```python
from build123d import *

# Parameters (mm, degrees)
F1_DEPTH = 30
F2_R     = 4.4
F3_R     = 4.4
F4_DEPTH = 25
F5_R     = 2
F6_R     = 2


# Not quite as in the source:
# - a feature names something its author has since deleted; it is built from what else it names


with BuildPart() as f1:
    # F0 (on Front) → F1 (new body)
    with BuildSketch(Plane.XZ):
        Polygon((90, -1), (90, 1), (70, 1), (70, 34), (-70, 34), (-70, 1), (-90, 1), (-90, -1), (-68, -1), (-68, 32), (68, 32), (68, -1), align=None)
    extrude(amount=F1_DEPTH)

    # F2 (on face) + F3 (on face) → F4 (cut)
    with BuildSketch(Plane.XY.offset(1)):
        with Locations((-80, -15)):
            Circle(F2_R)
        with Locations((80, -15)):
            Circle(F2_R)
    with BuildSketch(Plane.XY.offset(34)):
        with Locations((-25, -15)):
            Circle(F3_R)
        with Locations((25, -15)):
            Circle(F3_R)
    extrude(amount=-F4_DEPTH, mode=Mode.SUBTRACT)

    # F5
    f5_edges = [f1.edges().sort_by_distance(p)[0] for p in [
        (-70, -15, 34),
        (70, -15, 34),
    ]]
    fillet(f5_edges, radius=F5_R)

    # F6
    f6_edges = [f1.edges().sort_by_distance(p)[0] for p in [
        (68, -15, -1),
        (-68, -15, -1),
    ]]
    fillet(f6_edges, radius=F6_R)


solid = f1.part
```
The model under review builds one solid part; all positions refer to its coordinate system, in mm. A direction names the side the tool comes from. Round coordinates to 2 decimals unless told otherwise and drop trailing zeros. Order: outer loops, then holes, each group sorted by start corner. A loop starts at its lowest first (then second) coordinate and runs counter-clockwise, first axis right, second up.
(1) Take a section at C-C, the plane y = -7.75. State the section outline as (x, z) points, plus the area to 3 significant figures.
Working result:
outline: (-90, -1) - (-70, -1) arc R2 ccw to (-68, 1) - (-68, 32) - (68, 32) - (68, 1) arc R2 ccw to (70, -1) - (90, -1) - (90, 1) - (70, 1) - (70, 32) arc R2 ccw to (68, 34) - (-68, 34) arc R2 ccw to (-70, 32) - (-70, 1) - (-90, 1) - close
area: 489 mm2
(2) Take a section at B-B, the plane z = 12.5. State the section outline as (x, y) points.
Working result:
outline: (-70, -30) - (-68, -30) - (-68, 0) - (-70, 0) - close; (68, -30) - (70, -30) - (70, 0) - (68, 0) - close
(3) Tool access review of faces 4 (the face through (85, -15, 1)), 5 (the face through (-85, -15, -1)), 6 (the face through (27.365, -11.29, 33.014)), 7 (the face through (-75, -15, 1)), 8 (the face through (-1, -15, 32)): name each direction out of +Z, -Z, +X, -X, +Y, -Y from which nothing blocks a thin tool from reaching the whole face with its end or side.
Working result:
face 4: +Z, +X, +Y, -Y
face 5: -Z, +X, -X, +Y, -Y
face 6: +Z, -Z
face 7: +Z, -X, +Y, -Y
face 8: -Z, +Y, -Y
(4) Mouldability with a two-part tool opening along Y and no side actions: class faces 1 (the face through (70, -15, 16)), 2 (the face through (0, -30, 33)), 3 (the face through (75.604, -14.807, 0.014)) as released by +Y, released by -Y, zero draft, split by the parting line, or undercut.
Working result:
face 1: zero draft
face 2: released by -Y
face 3: undercut
(5) Wall thickness on L1, parallel to Y at x = 25, z = 33.05; L2, parallel to X at y = -5.5, z = 28.5; L3, parallel to X at y = -12.5, z = 32.5: over which ranges is each line inside the solid? List them lowest first.
Working result:
L1: y = -30 to -19.4, -10.6 to 0
L2: x = -70 to -68, 68 to 70
L3: x = -69.94 to -28.62, -21.38 to 21.38, 28.62 to 69.94
(6) For P1, Ø6, axis at y = -6.5, z = 29, coming from the +X side; P2, Ø5, axis at x = 49, y = -14, coming from the -Z side; P3, Ø10, axis at x = -80, y = -15, coming from the +Z side, all flat-tipped, find the tip position at first contact; note any pin that passes through.
Working result:
P1: stops at x = 70
P2: stops at z = 32
P3: stops at z = 1
(7) Take a section at D-D, the plane x = 7.5. State the section outline as (y, z) points, plus the area to 3 significant figures.
Working result:
outline: (-30, 32) - (0, 32) - (0, 34) - (-30, 34) - close
area: 60.0 mm2
(8) Take a section at A-A, the plane x = -80. State the section outline as (y, z) points.
Working result:
outline: (-30, -1) - (-19.4, -1) - (-19.4, 1) - (-30, 1) - close; (-10.6, -1) - (0, -1) - (0, 1) - (-10.6, 1) - close
